Geometry check sheet. Reference: drawing and pictorial views, mm from the part's lowest x, y, z. A direction names the side the tool comes from. Coordinates: 2 decimals unless noted, no trailing zeros. Loops run counter-clockwise (first coordinate to the right, second up) from the corner with the lowest first, then second, coordinate; pieces in that order, holes last. Notation, with made-up numbers: (11.5, -25.75) -> (42.5, -25.75) arc R34 ccw to (42.5, 10.25) -> close; hole circle Ø11 at (77.5, 46.25). An arc over 180 degrees is marked (long way). Answer as a JSON object with one key per item and string values. Group by question number.
Q1. Gauge pin test, flat ends, axial feed: pin 1 Ø1.5 at (x, z) = (2.5, 1) entering from -Y; pin 2 Ø1.5 at (x, z) = (2.5, 0.5) entering from +Y (1 decimal). Record the tip position at first contact, or that the pin passes through.
Q2. Scan lines: L1, parallel to X at y = 1.6, z = 3 (1 decimal); L2, parallel to Z at x = 0.5, y = 2.5 (1 decimal); L3, parallel to Z at x = 1.5, y = 1.85 (1 decimal). Record each from-to range of solid material in increasing order.
Q3. Set-up check for the marked faces 5 and 6: record each of +Z, -Z, +X, -X, +Y, -Y from which the full face is reachable in a straight line by a thin tool's end or side.
Q4. Release check for a two-part mould opening along Y. For the marked faces 1, 2, 3 and 4 record: released by +Y, released by -Y, zero draft, split by the parting line, or undercut.
Q5. Cross-section at A-A on x = 5. Record the boundary of the cut face in (y, z) (1 decimal).
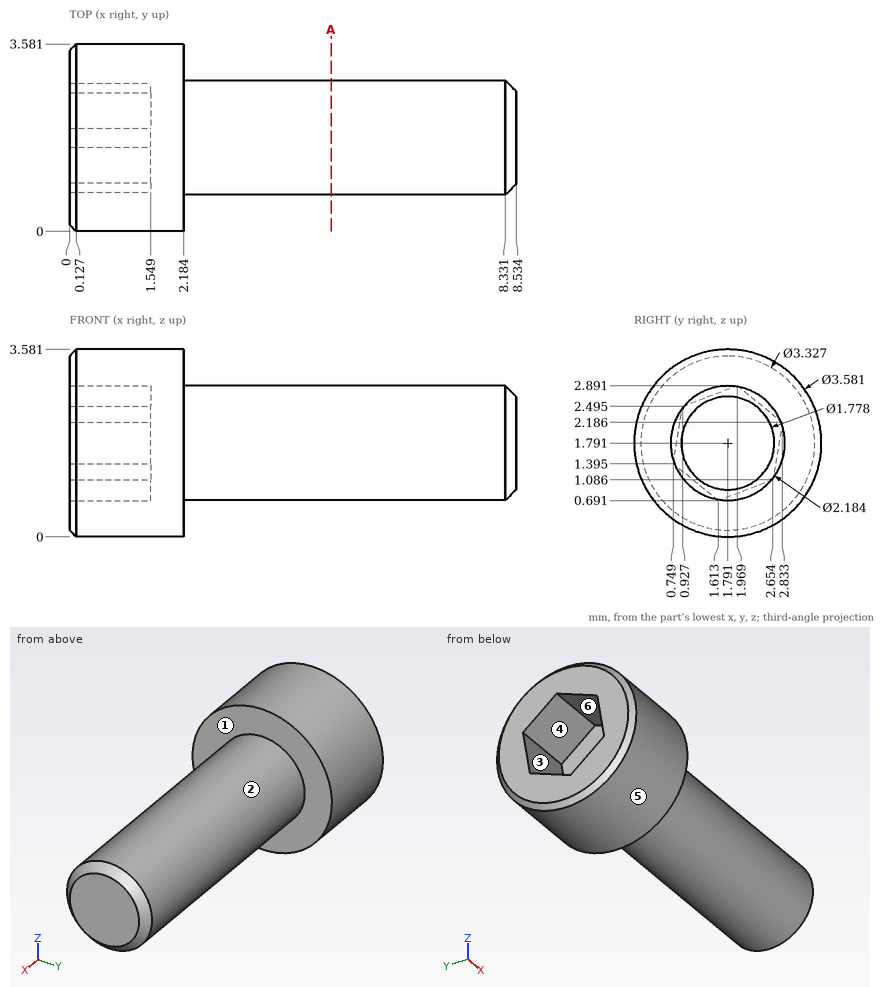
Computed values:
{
 "1": {"pin 1": "stops at y = 0", "pin 2": "stops at y = 3.5"},
 "2": {"L1": "x = 0 to 2.2", "L2": "z = 0.1 to 1, 2.5 to 3.4", "L3": "z = 0 to 0.8, 2.8 to 3.6"},
 "3": {"face 5": "+X, -X", "face 6": "-X"},
 "4": {"face 1": "zero draft", "face 2": "split by the parting line", "face 3": "undercut", "face 4": "undercut"},
 "5": {"outline": "circle Ø2.2 at (1.8, 1.8)"}
}
